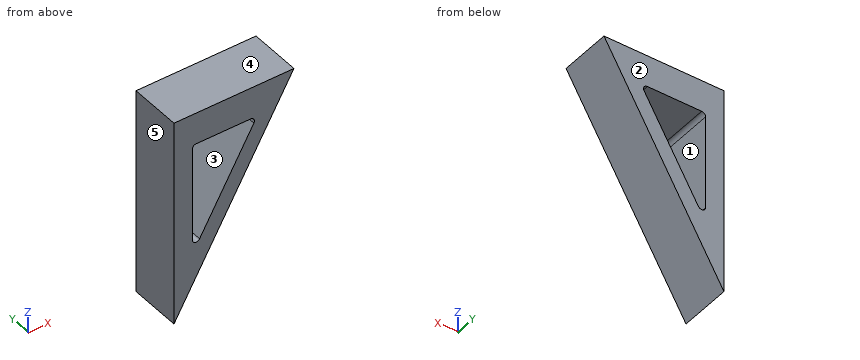
```python
from build123d import *

# Parameters (mm, degrees)
BOSS_EXTRUDE1_DEPTH = 20
CUT_EXTRUDE1_DEPTH  = 21
FILLET1_R           = 1.5


with BuildPart() as part:
    # Sketch1 → Boss-Extrude1 (new body)
    with BuildSketch(Plane(origin=(0, 0, 0), x_dir=(1, 0, 0), z_dir=(0, 1, 0))):
        Polygon((0, 0), (0, 80), (46.188021535, 0), align=None)
    extrude(amount=BOSS_EXTRUDE1_DEPTH)

    # Sketch2 → Cut-Extrude1 (cut, through all)
    with BuildSketch(Plane(origin=(0, 20, 0), x_dir=(1, 0, 0), z_dir=(0, 1, 0))):
        Polygon((7.062673845, 55.534180126), (7.062673845, 12.232909937), (32.062673845, 12.232909937), align=None)
    extrude(amount=-CUT_EXTRUDE1_DEPTH, mode=Mode.SUBTRACT)

    # Fillet1
    fillet1_edges = [part.edges().sort_by_distance(p)[0] for p in [
        (7.062673845, 10, -55.534180126),
        (32.062673845, 10, -12.232909937),
        (7.062673845, 10, -12.232909937),
    ]]
    fillet(fillet1_edges, radius=FILLET1_R)


solid = part.part
```
The model under review builds one solid part; all positions refer to its coordinate system, in mm. Face numbers are marked on the shaded views. A direction names the side the tool comes from. Round coordinates to 2 decimals unless told otherwise and drop trailing zeros. Order: outer loops, then holes, each group sorted by start corner. A loop starts at its lowest first (then second) coordinate and runs counter-clockwise, first axis right, second up. Notation, with made-up numbers: (-16.75, -9) -> (6.25, -9) arc R11 ccw to (6.25, 4) -> close; hole circle Ø7 at (-4.5, 2). An arc over 180 degrees is marked (long way). One line per item, written item: value. Start each with the question number.
Q1. Wall thickness on line 1 (X direction, y = 12.75, z = -46.5); line 2 (Z direction, x = 19.5, y = 15.25) (3 decimals); line 3 (X direction, y = 19.25, z = -29.5): over which ranges is each line inside the solid? List them lowest first.
Q2. Machinability: for the marked faces 1 and 2, which of the approach directions +Z, -Z, +X, -X, +Y, -Y give a long, thin tool a straight path to every point of the face, cutting with its end or side? Answer none if there is none.
Q3. Clearance check with flat-ended pins moving along their axes: pin 1 Ø10 at (x, y) = (15, 5) entering from -Z; pin 2 Ø8 at (x, y) = (25.5, 16) entering from -Z; pin 3 Ø10 at (y, z) = (7.5, -30.5) entering from +X; pin 4 Ø3 at (x, z) = (22.5, -46.5) entering from -Y. State where each tip first meets the part, or that it passes through.
Q4. Mouldability with a two-part tool opening along X and no side actions: class the marked faces 3, 4 and 5 as released by +X, released by -X, zero draft, split by the parting line, or undercut.
Q5. Take a section at D-D (z = -8). Write out the cut boundary in (x, y).
Q6. Take a section at C-C (z = -33). Write out the cut boundary in (x, y).
Q7. Take a section at B-B (x = 26). Write out the cut boundary in (y, z), and give its area (3 significant figures).
Q8. Take a section at A-A (y = 10.75). Write out the cut boundary in (x, z).
Reported:
1. line 1: x = 0 to 7.06, 12.28 to 19.34
1. line 2: z = -46.225 to -33.992, -12.233 to 0
1. line 3: x = 0 to 7.06, 22.09 to 29.16
2. face 1: +Y, -Y
2. face 2: +Z, -Z, +X, -X, +Y
3. pin 1: stops at z = -62.68
3. pin 2: stops at z = -42.76
3. pin 3: stops at x = 31.47
3. pin 4: passes through
4. face 3: undercut
4. face 4: zero draft
4. face 5: released by -X
5. outline: (0, 0) -> (41.57, 0) -> (41.57, 20) -> (0, 20) -> close
6. outline: (0, 0) -> (7.06, 0) -> (7.06, 20) -> (0, 20) -> close; (20.07, 0) -> (27.14, 0) -> (27.14, 20) -> (20.07, 20) -> close
7. outline: (0, -34.97) -> (20, -34.97) -> (20, -22.73) -> (0, -22.73) -> close; (0, -12.23) -> (20, -12.23) -> (20, 0) -> (0, 0) -> close
7. area: 489 mm2
8. outline: (0, -80) -> (46.19, 0) -> (0, 0) -> close; hole (7.06, -49.94) arc R1.5 ccw to (9.86, -50.69) -> (30.76, -14.48) arc R1.5 ccw to (29.46, -12.23) -> (8.56, -12.23) arc R1.5 ccw to (7.06, -13.73) -> close
